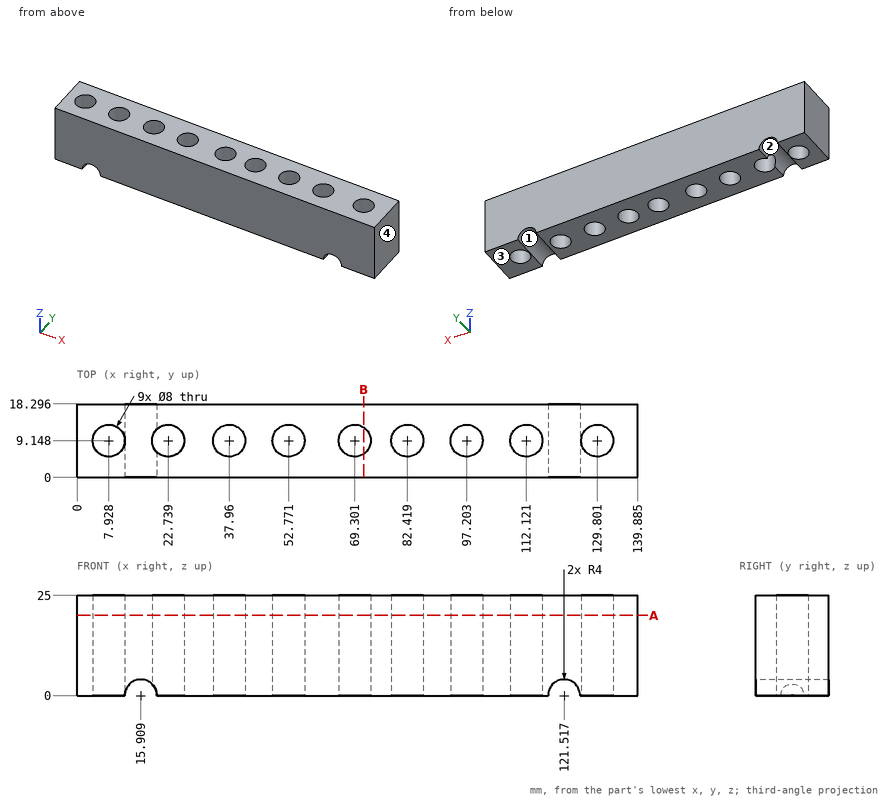
Input: dimensioned drawing with shaded views. Units: mm. Origin: part minimum x, y, z. Give positions to 0.01 mm unless a question says otherwise; leave off trailing zeros. Write each loop counter-clockwise with the first axis right and the second up, starting at its lowest first coordinate (ties: lowest second). Pieces come first, ordered by that corner, then holes. Notation, with made-up numbers: (40.25, 22.5) - (73.25, 22.5) arc R36 ccw to (73.25, 57.5) - close; hole circle Ø4 at (-39.75, 46). An arc over 180 degrees is marked (long way). One line per item, written item: value. Start each with the question number.
Q1. Draft query along X for the marked faces 1, 2, 3 and 4. Return one class per face: +X half, -X half, draft (parallel to the pull), parting line (faces both ways), or undercut.
Q2. Section query A-A, the plane z = 20. Count the separate pieces of the cut face and the enclosed holes in it, then the cut area to 3 significant figures.
Q3. Material intervals for probe 1 along Y at (x, z) = (84, 5.75) (1 decimal); probe 2 along Y at (x, z) = (96.5, 7.75) (1 decimal); probe 3 along Z at (x, y) = (18.5, 3.5), sorted ascending. Write a range as from..to.
Q4. First-contact query: pin 1 Ø7 at (x, y) = (22.74, 9.15) entering from -Z. Flat tip, straight axial feed; report the tip coordinate or a pass-through.
Q5. Section query B-B, the plane x = 71.5. Return the cut outline in (y, z).
Answer:
1. face 1: undercut
1. face 2: undercut
1. face 3: draft
1. face 4: +X half
2. separate pieces: 1
2. enclosed holes: 9
2. area: 2,110 mm2
3. probe 1: y = 0..5.5, 12.8..18.3
3. probe 2: y = 0..5.2, 13.1..18.3
3. probe 3: z = 3.05..25
4. pin 1: passes through
5. outline: (0, 0) - (5.81, 0) - (5.81, 25) - (0, 25) - close; (12.49, 0) - (18.3, 0) - (18.3, 25) - (12.49, 25) - close
